```python
from build123d import *

# Parameters (mm, degrees)
BOSS_EXTRUDE1_DEPTH = 9.525
FILLET1_R           = 3.175
BOSS_EXTRUDE2_DEPTH = 1.5875
SKETCH3_R           = 1.5875
CUT_EXTRUDE1_DEPTH  = 3.175
CHAMFER1_SIZE       = 1.5875
FILLET2_R           = 1.5875
CUT_EXTRUDE2_DEPTH  = 12.7
FILLET3_R           = 1.5875
SKETCH5_R           = 6.35
SKETCH5_R_2         = 1.5875
BOSS_EXTRUDE3_DEPTH = 3.175


with BuildPart() as part:
    # Sketch1 → Boss-Extrude1 (new body, symmetric)
    with BuildSketch(Plane.XY):
        Polygon((-0.3175, -0.3175), (-0.3175, 25.7175), (1.3335, 25.7175), (1.3335, 22.225), (4.191, 22.225), (4.191, 28.575), (1.016, 28.575), (-3.175, 28.575), (-3.175, 1.5875), (-12.7, 1.5875), (-12.7, -1.5875), (-3.175, -1.5875), (4.191, -1.5875), (4.191, 0), (4.191, 3.175), (1.3335, 3.175), (1.3335, -0.3175), align=None)
    extrude(amount=BOSS_EXTRUDE1_DEPTH, both=True)

    # Fillet1
    fillet1_edges = [part.edges().sort_by_distance(p)[0] for p in [
        (-3.175, 1.5875, 0),
    ]]
    fillet(fillet1_edges, radius=FILLET1_R)

    # Sketch2 → Boss-Extrude2 (add, symmetric)
    with BuildSketch(Plane.XY):
        Polygon((-3.175, 28.575), (-12.7, 1.5875), (-3.175, 1.5875), align=None)
    extrude(amount=BOSS_EXTRUDE2_DEPTH, both=True)

    # Sketch3 → Cut-Extrude1 (cut)
    with BuildSketch(Plane(origin=(0, 1.5875, 0), x_dir=(1, 0, 0), z_dir=(0, 1, 0))):
        with Locations((-9.525, -5.55625)):
            Circle(SKETCH3_R)
        with Locations((-9.525, 5.55625)):
            Circle(SKETCH3_R)
    extrude(amount=-CUT_EXTRUDE1_DEPTH, mode=Mode.SUBTRACT)

    # Chamfer1
    chamfer1_edges = [part.edges().sort_by_distance(p)[0] for p in [
        (4.191, 3.175, 0),
        (4.191, 22.225, 0),
    ]]
    chamfer(chamfer1_edges, length=CHAMFER1_SIZE)

    # Fillet2
    fillet2_edges = [part.edges().sort_by_distance(p)[0] for p in [
        (0.508, 28.575, -9.525),
        (0.508, 28.575, 9.525),
    ]]
    fillet(fillet2_edges, radius=FILLET2_R)

    # Sketch4 → Cut-Extrude2 (cut)
    with BuildSketch(Plane(origin=(0, 0, -1.5875), x_dir=(-1, 0, 0), z_dir=(0, 0, -1))):
        Polygon((12.7, 1.5875), (3.175, 28.575), (-4.191, 28.575), (-4.191, -1.5875), (12.7, -1.5875), align=None)
    extrude(amount=CUT_EXTRUDE2_DEPTH, mode=Mode.SUBTRACT)

    # Fillet3
    fillet3_edges = [part.edges().sort_by_distance(p)[0] for p in [
        (0.508, 28.575, -1.5875),
    ]]
    fillet(fillet3_edges, radius=FILLET3_R)

    # Sketch5 → Boss-Extrude3 (add)
    with BuildSketch(Plane(origin=(0, 1.5875, 0), x_dir=(1, 0, 0), z_dir=(0, 1, 0))):
        with Locations((-9.525, -5.55625)):
            Circle(SKETCH5_R)
        with Locations((-9.525, -5.55625)):
            Circle(SKETCH5_R_2, mode=Mode.SUBTRACT)
    extrude(amount=-BOSS_EXTRUDE3_DEPTH)


solid = part.part
```
Work out the finished part from the listing and answer in its coordinate system (mm). A direction names the side the tool comes from. Give positions to 0.01 mm unless a question says otherwise; leave off trailing zeros. Loops run counter-clockwise (first coordinate to the right, second up) from the corner with the lowest first, then second, coordinate; pieces in that order, holes last. Notation, with made-up numbers: (22, 46) - (68, 46) arc R28 cw to (68, 75) - close; hole circle Ø5 at (87.5, 68.25). An arc over 180 degrees is marked (long way). Use CSV: the item, a comma, the result in double quotes. Start each with the question number.
(1) Determine the mould class of faces 1 (the face through (-8.01, 0.02, 5.08)), 2 (the face through (0.28, 28.12, -1.11)), 3 (the face through (-7.87, 15.27, 0.02)), 4 (the face through (-6, 9, 1.588)) for opening direction Z: released by +Z, released by -Z, zero draft, split by the parting line, or undercut.
(2) Find section D-D, the plane x = -2.75. Determine the outline of the cut face in (y, z) (1 decimal).
(3) Find section A-A, the plane x = 0.5. Determine the outline of the cut face in (y, z) (1 decimal), plus the area to 3 significant figures.
(4) Find the intervals of material crossed by L1, parallel to Y at x = 0.75, z = 3.5 (1 decimal); L2, parallel to Z at x = -7.25, y = 13.5; L3, parallel to X at y = 16, z = 7.25 (1 decimal), in increasing order.
(5) Find section B-B, the plane y = 1. Count the separate pieces of the cut face and the enclosed holes in it, plus the area to 3 significant figures.
(6) A tool of negligible diameter and unlimited length cuts with its end or side. For faces 5 (the face through (3.39, 23.01, 3.89)), 6 (the face through (1.334, 1, 4)), 7 (the face through (-3.175, 17, 6)), 8 (the face through (-12.7, 0, -1)), from which of +Z, -Z, +X, -X, +Y, -Y can it reach the whole face along a straight path? Write none if from no direction.
(7) Each of these flat-tipped pins is pushed along its axis until it touches: pin 1 (5.5 mm diameter, centred on y = 14.5, z = 1.5, fed in from +X); pin 2 (3.5 mm diameter, centred on x = -12.5, z = 5, fed in from +Y); pin 3 (1 mm diameter, centred on x = -7.5, y = 7.5, fed in from +Z). Where does it stop, or does it pass through?
Results found:
1,face 1,"undercut"
1,face 2,"released by -Z"
1,face 3,"zero draft"
1,face 4,"released by +Z"
2,outline,"(-1.6, -1.6) - (27, -1.6) arc R1.6 ccw to (28.6, 0) - (28.6, 7.9) arc R1.6 ccw to (27, 9.5) - (-1.6, 9.5) - close"
3,outline,"(-1.6, -1.6) - (-0.3, -1.6) - (-0.3, 9.5) - (-1.6, 9.5) - close; (25.7, -1.6) - (27, -1.6) arc R1.6 ccw to (28.6, 0) - (28.6, 7.9) arc R1.6 ccw to (27, 9.5) - (25.7, 9.5) - close"
3,area,"44.8 mm^2"
4,L1,"-1.6 to -0.3, 25.7 to 28.6"
4,L2,"-1.59 to 1.59"
4,L3,"-3.2 to -0.3"
5,separate pieces,"2"
5,enclosed holes,"1"
5,area,"201 mm^2"
6,face 5,"+Z, -Z, +X"
6,face 6,"+Z, -Z"
6,face 7,"+Z, -X, +Y"
6,face 8,"-Z, -X, +Y, -Y"
7,pin 1,"x = -0.32"
7,pin 2,"y = 1.59"
7,pin 3,"z = 1.59"
